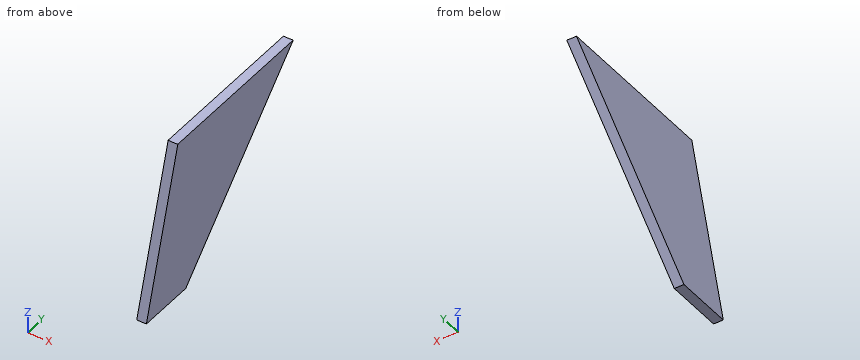
Autodesk Inventor part; units mm, degrees
ref_plane "YZ Plane" through (0, 0, 0) normal (1, 0, 0) x (0, 1, 0)
ref_plane "XZ Plane" through (0, 0, 0) normal (0, 1, 0) x (-1, 0, 0)
ref_plane "XY Plane" through (0, 0, 0) normal (0, 0, 1) x (1, 0, 0)
sketch "Sketch1" plane through (0, 0, 0) normal (1, 0, 0) x (0, 1, 0)
  line L0 (0, 0) -> (88, 0)
  line L1 (88, 0) -> (204.3575, 0) construction
  line L2 (88, 0) -> (6, -82)
  line L3 (88, 0) -> (171.4386, 0) construction
  line L4 (6, -82) -> (-24, -82)
  line L5 (-24, -82) -> (0, 0)
  dimension "d0" = 88
  dimension "d3" = 135
  dimension "d4" = 30
extrude "Extrusion1" add sketch "Sketch1" against normal blind 5
sketch "Sketch2" plane through (0, 0, 0) normal (0, 1, 0) x (-1, 0, 0)
  line L0 (0, 0) -> (5, 0)
  circle A0 centre (2.5, 0) radius 36.5
  line L1 (0, 0) -> (0, -82)
  circle A1 centre (2.5, 36.5) radius 36.5855
  line L2 (5, -82) -> (5, 0)
  line L3 (0, 0) -> (5, 0)
  dimension "d7" = 73
extrude "Extrusion2" cut sketch "Sketch2" along normal mid plane 197.25 contours L0 A1
properties part number "Aletas" material "Birch"
CAD build for the part. Positions are in the model's coordinates, mm. Round coordinates to 2 decimals unless told otherwise and drop trailing zeros. Order: outer loops, then holes, each group sorted by start corner. A loop starts at its lowest first (then second) coordinate and runs counter-clockwise, first axis right, second up.
Q1. Slice it at C-C (z = -33). Write the cut outline in (x, y).
Q2. Wall check: L1, parallel to Z at x = -1.8, y = 64; L2, parallel to Z at x = -4, y = 26; L3, parallel to Y at x = -3.7, z = -66. Give the ranges that are in metal, low to high.
Q3. Slice it at D-D (x = -4.2). Write the cut outline in (y, z), and give its area (3 significant figures).
Q4. Drop flat-ended pins along their axis: pin 1 (1 mm diameter, centred on x = -3, z = -51, fed in from +Y); pin 2 (1.5 mm diameter, centred on x = -0.5, y = 31.5, fed in from -Z). Give the stop position or say it passes through.
Results below:
1. outline: (-5, -9.66) - (0, -9.66) - (0, 55) - (-5, 55) - close
2. L1: z = -24 to -0.08
2. L2: z = -62 to -0.05
2. L3: y = -19.32 to 22
3. outline: (-24, -82) - (6, -82) - (87.95, -0.05) - (-0.01, -0.05) - close
3. area: 4,830 mm2
4. pin 1: stops at y = 37.5
4. pin 2: stops at z = -57.25
